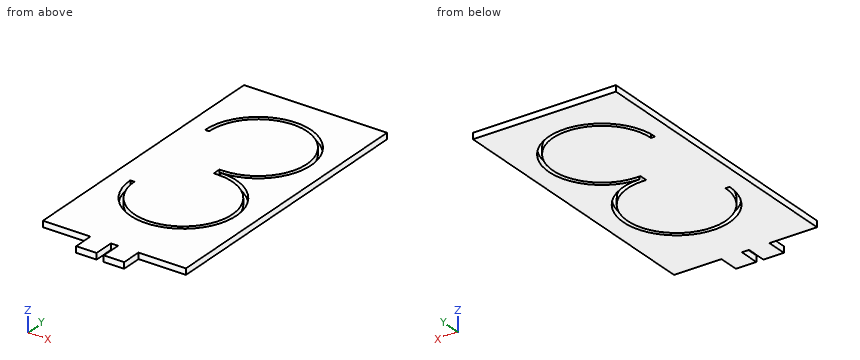
```python
from build123d import *

# Parameters (mm, degrees)
SKIZZE1_W                       = 35
SKIZZE1_H                       = 75
AUFSATZ_LINEAR_AUSTRAGEN1_DEPTH = 1.5
SKIZZE2_W                       = 11.63
SKIZZE2_H                       = 5
SKIZZE2_W_2                     = 11.62
SKIZZE2_W_3                     = 1.75
SCHNITT_LINEAR_AUSTRAGEN1_DEPTH = 1.5
SCHNITT_LINEAR_AUSTRAGEN4_DEPTH = 20


with BuildPart() as part:
    # Skizze1 → Aufsatz-Linear austragen1 (new body)
    with BuildSketch(Plane.XY):
        with Locations((17.5, 37.5)):
            Rectangle(SKIZZE1_W, SKIZZE1_H)
    extrude(amount=AUFSATZ_LINEAR_AUSTRAGEN1_DEPTH)

    # Skizze2 → Schnitt-Linear austragen1 (cut)
    with BuildSketch(Plane.XY.offset(1.5)):
        with Locations((5.815, 2.5)):
            Rectangle(SKIZZE2_W, SKIZZE2_H)
        with Locations((29.19, 2.5)):
            Rectangle(SKIZZE2_W_2, SKIZZE2_H)
        with Locations((17.505, 2.5)):
            Rectangle(SKIZZE2_W_3, SKIZZE2_H)
    extrude(amount=-SCHNITT_LINEAR_AUSTRAGEN1_DEPTH, mode=Mode.SUBTRACT)

    # Skizze9 → Schnitt-Linear austragen4 (cut)
    with BuildSketch(Plane.XY.offset(1.5)):
        with BuildLine():
            Line((5.5, 55), (4.5, 55))
            ThreePointArc((4.5, 55), (26.692388155, 64.192388155), (17.5, 42))
            ThreePointArc((17.5, 42), (26.692388155, 19.807611845), (4.5, 29))
            Line((4.5, 29), (5.5, 29))
            ThreePointArc((5.5, 29), (25.985281374, 20.514718626), (17.5, 41))
            Line((17.5, 41), (16.5, 41))
            Line((16.5, 41), (16.5, 43))
            Line((16.5, 43), (17.5, 43))
            ThreePointArc((17.5, 43), (25.985281374, 63.485281374), (5.5, 55))
        make_face()
    extrude(amount=-SCHNITT_LINEAR_AUSTRAGEN4_DEPTH, mode=Mode.SUBTRACT)


solid = part.part
```
For this review, take the finished solid that the model builds, in its own axes (mm). Give positions to 0.01 mm unless a question says otherwise; leave off trailing zeros. Write each loop counter-clockwise with the first axis right and the second up, starting at its lowest first coordinate (ties: lowest second). Pieces come first, ordered by that corner, then holes. Notation, with made-up numbers: M 31,46 L 41,46 A23 ccw 41,80 Z; hole C 15,50 d4. An arc over 180 degrees is marked long. Answer as a JSON object with one key per item and string values. Group by question number.
Item 1: Consider section A-A on z = 0.6. Write out the cut boundary in (x, y), plus the area to 3 significant figures.
Item 2: Consider section B-B on x = 26. Write out the cut boundary in (y, z).
Item 3: Consider section D-D on y = 33. Write out the cut boundary in (x, z).
Item 4: Consider section C-C on y = 18. Write out the cut boundary in (x, z).
Item 5: For pin 1 Ø0.8 at (x, z) = (26.5, 1) entering from -Y, flat-tipped, find the tip position at first contact; note if it passes through.
Item 6: For probe 1 along Y at (x, z) = (11, 0.5); probe 2 along Y at (x, z) = (7.5, 0.3); probe 3 along Y at (x, z) = (27, 0.4), list the stretches that pass through material, from the lowest coordinate up. Write a range as [from, to].
Check result:
{
 "1": {"outline": "M 0,5 L 11.63,5 L 11.63,0 L 16.63,0 L 16.63,5 L 18.38,5 L 18.38,0 L 23.38,0 L 23.38,5 L 35,5 L 35,75 L 0,75 Z; hole M 4.5,29 A13 ccw long 17.5,42 A13 ccw long 4.5,55 L 5.5,55 A12 cw long 17.5,43 L 16.5,43 L 16.5,41 L 17.5,41 A12 cw long 5.5,29 Z", "area": "2,380 mm^2"},
 "2": {"outline": "M 5,0 L 19.16,0 L 19.16,1.5 L 5,1.5 Z; M 20.53,0 L 37.47,0 L 37.47,1.5 L 20.53,1.5 Z; M 38.84,0 L 45.16,0 L 45.16,1.5 L 38.84,1.5 Z; M 46.53,0 L 63.47,0 L 63.47,1.5 L 46.53,1.5 Z; M 64.84,0 L 75,0 L 75,1.5 L 64.84,1.5 Z"},
 "3": {"outline": "M 0,0 L 28.81,0 L 28.81,1.5 L 0,1.5 Z; M 29.87,0 L 35,0 L 35,1.5 L 29.87,1.5 Z"},
 "4": {"outline": "M 0,0 L 10.57,0 L 10.57,1.5 L 0,1.5 Z; M 12.7,0 L 22.3,0 L 22.3,1.5 L 12.7,1.5 Z; M 24.43,0 L 35,0 L 35,1.5 L 24.43,1.5 Z"},
 "5": {"pin 1": "stops at y = 5"},
 "6": {"probe 1": "y = [5, 17.74], [18.91, 65.09], [66.26, 75]", "probe 2": "y = [5, 20.69], [22.37, 61.63], [63.31, 75]", "probe 3": "y = [5, 20.13], [21.67, 36.33], [37.87, 46.13], [47.67, 62.33], [63.87, 75]"}
}
